Design review of the part built by this model. Coordinates are the model's own, in mm. A direction names the side the tool comes from. Coordinates: 2 decimals unless noted, no trailing zeros. Use a Markdown table: item, result. Add a question column.
Q1. For probe 1 along Y at (x, z) = (608.5, -23.5); probe 2 along Z at (x, y) = (783, 175); probe 3 along X at (y, z) = (295.5, 96.5), list the stretches that pass through material, from the lowest coordinate up.
Q2. For faces 1 (the face through (915.757, 283.78, 3.425)), 2 (the face through (491, 550, 240)), list the 3-axis set-ups (+Z, -Z, +X, -X, +Y, -Y) from which the entire face can be reached by the end or side of a thin tool; tool diameter is ignored.
Q3. Clearance check with flat-ended pins moving along their axes: pin 1 Ø11 at (x, y) = (97.5, 128.5) entering from +Z; pin 2 Ø8 at (x, y) = (97.65, 130.88) entering from +Z; pin 3 Ø5 at (x, y) = (97, 131) entering from -Z. State where each tip first meets the part, or that it passes through.
Q4. Draft analysis for pull direction Z (two halves, no side actions). For faces 3 (the face through (456, 0, -15)), 4 (the face through (10, 284, -3)), state which applies: pulls with the +Z half, pulls with the -Z half, needs draft (parallel to the pull), parting line crosses it, or undercut.
from build123d import *

# Parameters (mm, degrees)
CASCA4_T                = -10
CUT_EXTRUDE3_DEPTH      = 23
CUT_EXTRUDE3_DEPTH_BACK = 452
SKETCH3_R               = 5
CUT_EXTRUDE4_DEPTH      = 8
CUT_EXTRUDE4_DEPTH_BACK = 439
SKETCH4_R               = 5
SKETCH5_R               = 5
CUT_EXTRUDE5_DEPTH      = 55
SKETCH6_R               = 5
CUT_EXTRUDE6_DEPTH      = 56
SKETCH8_R               = 5
CUT_EXTRUDE7_DEPTH      = 20
SKETCH9_R               = 5
CUT_EXTRUDE8_DEPTH      = 20


with BuildPart() as part:
    # Esboço1 → Loft3 section 0
    with BuildSketch(Plane(origin=(0, 0, 0), x_dir=(1, 0, 0), z_dir=(0, 1, 0))):
        with BuildLine():
            Line((0, 225), (0, -225))
            Line((0, -225), (900, -247.5))
            Line((900, -247.5), (900, 247.5))
            Line((900, 247.5), (0, 225))
        make_face()
    # Esboço2 → Loft3 section 1
    with BuildSketch(Plane(origin=(0, 550, 0), x_dir=(1, 0, 0), z_dir=(0, 1, 0))):
        with BuildLine():
            Line((0, 225), (0, -225))
            Line((0, -225), (950, -255))
            Line((950, -255), (950, 255))
            Line((950, 255), (0, 225))
        make_face()
    loft()

    # Casca4
    casca4_openings = [part.faces().sort_by_distance(p)[0] for p in [
        (484.895833333, 550, 0),
    ]]
    offset(amount=CASCA4_T, openings=casca4_openings, kind=Kind.INTERSECTION)

    # Cut-Extrude1: read off the stored shape, not the designer's step
    # Cut-Extrude1: loft between two sections, ruled curve by curve
    cut_extrude1_from = [
        Edge.make_three_point_arc((121.101758385, 525.076407947, -225), (116.101758385, 530.076407947, -225), (111.101758385, 525.076407947, -225)),
        Edge.make_three_point_arc((111.101758385, 525.076407947, -225), (116.101758385, 520.076407947, -225), (121.101758385, 525.076407947, -225)),
    ]
    cut_extrude1_to = [
        Edge.make_three_point_arc((121.101758385, 525.076407947, -218.471984374), (116.101758385, 530.076407947, -218.471984374), (111.101758385, 525.076407947, -218.471984374)),
        Edge.make_three_point_arc((111.101758385, 525.076407947, -218.471984374), (116.101758385, 520.076407947, -218.471984374), (121.101758385, 525.076407947, -218.471984374)),
    ]
    cut_extrude1 = Solid(Shell([*[Face.make_surface_from_curves(cut_extrude1_from[k], cut_extrude1_to[k]) for k in range(2)], Face(Wire(cut_extrude1_from)), Face(Wire(cut_extrude1_to))]))
    add(cut_extrude1, mode=Mode.SUBTRACT)

    # Cut-Extrude1 2: loft between two sections, ruled curve by curve
    cut_extrude1_2_from = [
        Edge.make_three_point_arc((121.101758385, 525.076407947, 218.471984384), (116.101758385, 530.076407947, 218.471984384), (111.101758385, 525.076407947, 218.471984384)),
        Edge.make_three_point_arc((111.101758385, 525.076407947, 218.471984384), (116.101758385, 520.076407947, 218.471984384), (121.101758385, 525.076407947, 218.471984384)),
    ]
    cut_extrude1_2_to = [
        Edge.make_three_point_arc((121.101758385, 525.076407947, 225), (116.101758385, 530.076407947, 225), (111.101758385, 525.076407947, 225)),
        Edge.make_three_point_arc((111.101758385, 525.076407947, 225), (116.101758385, 520.076407947, 225), (121.101758385, 525.076407947, 225)),
    ]
    cut_extrude1_2 = Solid(Shell([*[Face.make_surface_from_curves(cut_extrude1_2_from[k], cut_extrude1_2_to[k]) for k in range(2)], Face(Wire(cut_extrude1_2_from)), Face(Wire(cut_extrude1_2_to))]))
    add(cut_extrude1_2, mode=Mode.SUBTRACT)

    # Cut-Extrude2: read off the stored shape, not the designer's step
    # Cut-Extrude2: loft between two sections, ruled curve by curve
    cut_extrude2_from = [
        Edge.make_three_point_arc((822.470918457, 525.465412678, -247), (817.470918457, 530.465412678, -247), (812.470918457, 525.465412678, -247)),
        Edge.make_three_point_arc((812.470918457, 525.465412678, -247), (817.470918457, 520.465412678, -247), (822.470918457, 525.465412678, -247)),
    ]
    cut_extrude2_to = [
        Edge.make_three_point_arc((822.470918457, 525.465412678, -240.418518829), (817.470918457, 530.465412678, -240.418518829), (812.470918457, 525.465412678, -240.418518829)),
        Edge.make_three_point_arc((812.470918457, 525.465412678, -240.418518829), (817.470918457, 520.465412678, -240.418518829), (822.470918457, 525.465412678, -240.418518829)),
    ]
    cut_extrude2 = Solid(Shell([*[Face.make_surface_from_curves(cut_extrude2_from[k], cut_extrude2_to[k]) for k in range(2)], Face(Wire(cut_extrude2_from)), Face(Wire(cut_extrude2_to))]))
    add(cut_extrude2, mode=Mode.SUBTRACT)

    # Cut-Extrude2 2: loft between two sections, ruled curve by curve
    cut_extrude2_2_from = [
        Edge.make_three_point_arc((822.470918457, 525.465412678, 240.418519067), (817.470918457, 530.465412678, 240.418519067), (812.470918457, 525.465412678, 240.418519067)),
        Edge.make_three_point_arc((812.470918457, 525.465412678, 240.418519067), (817.470918457, 520.465412678, 240.418519067), (822.470918457, 525.465412678, 240.418519067)),
    ]
    cut_extrude2_2_to = [
        Edge.make_three_point_arc((822.470918457, 525.465412678, 247), (817.470918457, 530.465412678, 247), (812.470918457, 525.465412678, 247)),
        Edge.make_three_point_arc((812.470918457, 525.465412678, 247), (817.470918457, 520.465412678, 247), (822.470918457, 525.465412678, 247)),
    ]
    cut_extrude2_2 = Solid(Shell([*[Face.make_surface_from_curves(cut_extrude2_2_from[k], cut_extrude2_2_to[k]) for k in range(2)], Face(Wire(cut_extrude2_2_from)), Face(Wire(cut_extrude2_2_to))]))
    add(cut_extrude2_2, mode=Mode.SUBTRACT)

    # Sketch3 → Cut-Extrude3 (cut, two sides: drawn at the far end of the back side and taken through both)
    with BuildSketch(Plane.XY.offset(215).offset(-CUT_EXTRUDE3_DEPTH_BACK)):
        with Locations((529.096415143, 195.085241143)):
            Circle(SKETCH3_R)
    extrude(amount=CUT_EXTRUDE3_DEPTH + CUT_EXTRUDE3_DEPTH_BACK, mode=Mode.SUBTRACT)

    # Sketch4 → Cut-Extrude4 (cut, two sides: drawn at the far end of the back side and taken through both)
    with BuildSketch(Plane.XY.offset(215).offset(-CUT_EXTRUDE4_DEPTH_BACK)):
        with Locations((97.648591279, 130.881920188)):
            Circle(SKETCH4_R)
    extrude(amount=CUT_EXTRUDE4_DEPTH + CUT_EXTRUDE4_DEPTH_BACK, mode=Mode.SUBTRACT)

    # Sketch5 → Cut-Extrude5 (cut)
    with BuildSketch(Plane(origin=(890, 0, 0), x_dir=(0, 0, -1), z_dir=(1, 0, 0))):
        with Locations(Location((175.040186522, 523.527338852, 0), (0, 0, 270))):
            Circle(SKETCH5_R)
    extrude(amount=CUT_EXTRUDE5_DEPTH, mode=Mode.SUBTRACT)

    # Sketch6 → Cut-Extrude6 (cut)
    with BuildSketch(Plane(origin=(890, 0, 0), x_dir=(0, 0, -1), z_dir=(1, 0, 0))):
        with Locations(Location((-174.853977213, 523.054329593, 0), (0, 0, 270))):
            Circle(SKETCH6_R)
    extrude(amount=CUT_EXTRUDE6_DEPTH, mode=Mode.SUBTRACT)

    # Sketch8 → Cut-Extrude7 (cut)
    with BuildSketch(Plane(origin=(890, 0, 0), x_dir=(0, 0, -1), z_dir=(1, 0, 0))):
        with Locations(Location((173.846443874, 154.777832346, 0), (0, 0, 270))):
            Circle(SKETCH8_R)
    extrude(amount=CUT_EXTRUDE7_DEPTH, mode=Mode.SUBTRACT)

    # Sketch9 → Cut-Extrude8 (cut)
    with BuildSketch(Plane(origin=(890, 0, 0), x_dir=(0, 0, -1), z_dir=(1, 0, 0))):
        with Locations(Location((-164.798644624, 157.991483325, 0), (0, 0, 270))):
            Circle(SKETCH9_R)
    extrude(amount=CUT_EXTRUDE8_DEPTH, mode=Mode.SUBTRACT)


solid = part.part
Answer list:
| question | item | result |
|---|---|---|
| 1 | probe 1 | 0 to 10 |
| 1 | probe 2 | -246.28 to -236.27, 236.27 to 246.28 |
| 1 | probe 3 | 0 to 10, 916.82 to 926.86 |
| 2 | face 1 | +Y |
| 2 | face 2 | +Z, -Z, +X, -X, +Y |
| 3 | pin 1 | z = 227.74 |
| 3 | pin 2 | z = 227.71 |
| 3 | pin 3 | z = -227.65 |
| 4 | face 3 | needs draft |
| 4 | face 4 | undercut |
